Geometry check sheet. Reference: the model listing, model coordinates, mm. Give positions to 0.01 mm unless a question says otherwise; leave off trailing zeros. Loops run counter-clockwise (first coordinate to the right, second up) from the corner with the lowest first, then second, coordinate; pieces in that order, holes last. Notation, with made-up numbers: (-31.75, 79.25) -> (4.25, 79.25) arc R21 cw to (4.25, 86.25) -> close; hole circle Ø2 at (-24.5, 59.5). An arc over 180 degrees is marked (long way). One line per item, written item: value. Start each with the question number.
(1) Gauge pin test, flat ends, axial feed: pin 1 Ø1.5 at (x, z) = (-6, -4.5) entering from +Y; pin 2 Ø1.5 at (y, z) = (-22, -3.5) entering from -X. Record the tip position at first contact, or that the pin passes through.
(2) Sectioned sample at B-B, the plane z = -1.25. State how many separate pieces and enclosed holes the cut face has, then the cut area to 3 significant figures.
(3) Sectioned sample at C-C, the plane x = 31.75. Record the cut outline in (y, z).
(4) Draft check along Y on faces 1 (the face through (34.242, 0.553, -3.219)), 2 (the face through (36.85, 4.11, -3.13)), 3 (the face through (26.78, -27.38, -3.13)). Enter one of: pulls with the +Y half, pulls with the -Y half, needs draft (parallel to the pull), parting line crosses it, or undercut.
(5) Sectioned sample at A-A, the plane y = -31.75. Record the cut outline in (x, z).
(6) Scan lines: line 1 along Y through (x, z) = (0, -2.5) (3 decimals); line 2 along X through (y, z) = (-31, -2.25); line 3 along X through (y, z) = (3, -6). Record each from-to range of solid material in increasing order. Write a range as from..to.
(7) Sectioned sample at D-D, the plane y = -25. Record the cut outline in (x, z).
Autodesk Inventor part; units mm, degrees
ref_plane "YZ Plane" through (0, 0, 0) normal (1, 0, 0) x (0, 1, 0)
ref_plane "XZ Plane" through (0, 0, 0) normal (0, 1, 0) x (-1, 0, 0)
ref_plane "XY Plane" through (0, 0, 0) normal (0, 0, 1) x (1, 0, 0)
sketch "Sketch1" plane through (0, 0, 0) normal (0, 0, 1) x (1, 0, 0)
  circle A0 centre (0, 0) radius 31.75 construction
  circle A1 centre (0, 0) radius 11.176 construction
  line L0 (0, 0) -> (17.9605, -17.9605) construction
  line L1 (0, 0) -> (0, -31.75) construction
  circle A2 centre (17.9605, -17.9605) radius 6.55 construction
  circle A3 centre (0, 31.75) radius 6.55 construction
  circle A4 centre (0, -31.75) radius 6.55 construction
  circle A5 centre (31.75, 0) radius 6.55 construction
  circle A6 centre (-31.75, 0) radius 6.55 construction
  circle A7 centre (0, 0) radius 25.2 construction
  circle A8 centre (0, 0) radius 38.3 construction
  arc A9 (0, -25.2) -> (12.6501, -21.7948) centre (0, 0) ccw
  arc A10 (0, -25.2) -> (0, -38.3) centre (0, -31.75) ccw
  arc A11 (0, -38.3) -> (38.3, 0) centre (0, 0) ccw
  arc A12 (38.3, 0) -> (25.2, 0) centre (31.75, 0) ccw
  arc A13 (21.7948, -12.6501) -> (25.2, 0) centre (0, 0) ccw
  arc A14 (21.7948, -12.6501) -> (12.6501, -21.7948) centre (17.9605, -17.9605) ccw
  dimension "d0" = 63.5
  dimension "d1" = 22.352
  dimension "d3" = 25.4
  dimension "d4" = 45
  dimension "d5" = 13.1
  dimension "d6" = 13.1
  dimension "d7" = 13.1
  dimension "d8" = 13.1
  dimension "d9" = 13.1
  dimension "d10" = 6.55
  dimension "d11" = 13.1
extrude "Extrusion1" add sketch "Sketch1" against normal blind 6.35
hole "Hole1" at (0, 31.75, 0) at (17.9605, -17.9605, 0) direction (0, 0, -1) diameter 6.75 depth 9.525
sketch "Sketch2" plane through (0, 0, 0) normal (0, 0, 1) x (1, 0, 0)
  circle A0 centre (17.9605, -17.9605) radius 3.375 construction
  arc A1 (21.7948, -12.6501) -> (25.2, 0) centre (0, 0) ccw
  arc A2 (38.3, 0) -> (25.2, 0) centre (31.75, 0) ccw
  arc A3 (0, -38.3) -> (38.3, 0) centre (0, 0) ccw construction
  arc A4 (0, -25.2) -> (0, -38.3) centre (0, -31.75) ccw
  arc A5 (0, -25.2) -> (12.6501, -21.7948) centre (0, 0) ccw
  arc A6 (21.7948, -12.6501) -> (12.6501, -21.7948) centre (17.9605, -17.9605) ccw
  circle A7 centre (0, 0) radius 12.7
  line L0 (-12.4595, -2.46) -> (-6.4259, -33.0187)
  arc A8 (0, -25.2) -> (0, -38.3) centre (0, -31.75) ccw construction
  line L1 (2.46, 12.4595) -> (33.0187, 6.4259)
  circle A9 centre (0, 0) radius 9.525
  dimension "d23" = 3.175
  dimension "d24" = 19.05
extrude "Extrusion2" add sketch "Sketch2" against normal blind 6.35
hole "Hole2" at (0, -31.75, 0) at (31.75, 0, 0) direction (0, 0, -1) diameter 5.1054 depth 9.525
equation "\"d6\" = d5"
equation "\"d7\" = d5"
equation "\"d8\" = d5"
equation "\"d9\" = d5"
equation "\"d10\" = 0.5 * d5"
equation "\"d11\" = d5"
properties part number "CL7-018" material "ABS Plastic"
Calculated:
1. pin 1: stops at y = 11.56
1. pin 2: stops at x = -8.75
2. separate pieces: 1
2. enclosed holes: 4
2. area: 1,610 mm2
3. outline: (-21.42, -6.35) -> (-2.55, -6.35) -> (-2.55, 0) -> (-21.42, 0) -> close; (2.55, -6.35) -> (6.68, -6.35) -> (6.68, 0) -> (2.55, 0) -> close
4. face 1: undercut
4. face 2: pulls with the +Y half
4. face 3: pulls with the -Y half
5. outline: (-6.68, -6.35) -> (-2.55, -6.35) -> (-2.55, 0) -> (-6.68, 0) -> close; (2.55, -6.35) -> (21.42, -6.35) -> (21.42, 0) -> (2.55, 0) -> close
6. line 1: y = -38.3..-34.303, -29.197..-9.525, 9.525..12.7
6. line 2: x = -6.82..-2.44, 2.44..22.49
6. line 3: x = -12.34..-9.04, 9.04..37.57
7. outline: (-8.01, -6.35) -> (29.02, -6.35) -> (29.02, 0) -> (-8.01, 0) -> close
